```python
from build123d import *

# Parameters (mm, degrees)
SKETCH_1_R          = 7
EXTRUDE_1_DEPTH     = 2
SKETCH_2_W          = 16
SKETCH_2_H          = 16
EXTRUDE_2_DEPTH     = 18
SKETCH_3_W          = 8
SKETCH_3_H          = 16
CUT_EXTRUDE_1_DEPTH = 16
CUT_EXTRUDE_2_DEPTH = 16


with BuildPart() as part:
    # 草图1 → 凸台-拉伸1 (new body)
    with BuildSketch(Plane(origin=(0, 0, 0), x_dir=(1, 0, 0), z_dir=(0, 1, 0))):
        Circle(SKETCH_1_R)
    extrude(amount=EXTRUDE_1_DEPTH)

    # 草图2 → 凸台-拉伸2 (add)
    with BuildSketch(Plane(origin=(0, 2, 0), x_dir=(1, 0, 0), z_dir=(0, 1, 0))):
        Rectangle(SKETCH_2_W, SKETCH_2_H)
    extrude(amount=EXTRUDE_2_DEPTH)

    # 草图3 → 切除-拉伸1 (cut)
    with BuildSketch(Plane.XY.offset(8)):
        with Locations((0, 12)):
            Rectangle(SKETCH_3_W, SKETCH_3_H)
    extrude(amount=-CUT_EXTRUDE_1_DEPTH, mode=Mode.SUBTRACT)

    # 草图4 → 切除-拉伸2 (cut)
    with BuildSketch(Plane(origin=(8, 0, 0), x_dir=(0, 0, -1), z_dir=(1, 0, 0))):
        with BuildLine():
            Line((-8, 12), (-8, 21.557868838))
            Line((-8, 21.557868838), (8, 21.557868838))
            Line((8, 21.557868838), (8, 12))
            ThreePointArc((8, 12), (0, 20), (-8, 12))
        make_face()
    extrude(amount=-CUT_EXTRUDE_2_DEPTH, mode=Mode.SUBTRACT)


solid = part.part
```
The listing builds one solid part. Answer for the finished solid, in the listing's coordinates (mm). A direction names the side the tool comes from. Give positions to 0.01 mm unless a question says otherwise; leave off trailing zeros. Order: outer loops, then holes, each group sorted by start corner. A loop starts at its lowest first (then second) coordinate and runs counter-clockwise, first axis right, second up.
1) Find section D-D on z = -4. Write down the section's boundary in (x, y), then the cut area to 3 significant figures.
Reported:
outline: (-8, 2) - (-5.74, 2) - (-5.74, 0) - (5.74, 0) - (5.74, 2) - (8, 2) - (8, 18.93) - (4, 18.93) - (4, 4) - (-4, 4) - (-4, 18.93) - (-8, 18.93) - close
area: 174 mm2
2) Consider line 1 along X through (y, z) = (16.5, -1.5); line 2 along Y through (x, z) = (0, 3.75); line 3 along Y through (x, z) = (-3.5, 6.5). Determine where each line is inside the solid, lowest interval first.
Reported:
line 1: x = -8 to -4, 4 to 8
line 2: y = 0 to 4
line 3: y = 2 to 4
3) Find section A-A on y = 13.75. Write down the section's boundary in (x, z).
Reported:
outline: (-8, -7.81) - (-4, -7.81) - (-4, 7.81) - (-8, 7.81) - close; (4, -7.81) - (8, -7.81) - (8, 7.81) - (4, 7.81) - close
4) Find section C-C on x = -0.75. Write down the section's boundary in (y, z), then the cut area to 3 significant figures.
Reported:
outline: (0, -6.96) - (2, -6.96) - (2, -8) - (4, -8) - (4, 8) - (2, 8) - (2, 6.96) - (0, 6.96) - close
area: 59.8 mm2
5) Determine the mould class of faces 4 (the face through (4, 12, 0)), 5 (the face through (-0.1, 3.6, 8)), 6 (the face through (0, 4, 0)), 7 (the face through (8, 11, 0)) for opening direction X: pulls with the +X half, pulls with the -X half, needs draft (parallel to the pull), parting line crosses it, or undercut.
Reported:
face 4: undercut
face 5: needs draft
face 6: undercut
face 7: pulls with the +X half
6) For faces 1 (the face through (6, 20, 0)), 2 (the face through (-4, 12, 0)), 3 (the face through (6.466, 0.986, 2.681)), determine the directions among +Z, -Z, +X, -X, +Y, -Y from which every point of the face is accessible in a straight line to the end or side of a thin tool.
Reported:
face 1: +X, -X, +Y
face 2: +Z, -Z, +Y
face 3: -Y
7) Given P1, Ø2, axis at x = -5, z = 3.5, coming from the -Y side; P2, Ø6.5, axis at x = 0, z = -1.5, coming from the +Y side; P3, Ø1, axis at x = -2.5, y = 11.5, coming from the -Z side, each flat-ended and moving along its own axis, determine where each tip first touches the part or whether it passes through.
Reported:
P1: stops at y = 0
P2: stops at y = 4
P3: passes through
8) Find section B-B on z = 0. Write down the section's boundary in (x, y).
Reported:
outline: (-8, 2) - (-7, 2) - (-7, 0) - (7, 0) - (7, 2) - (8, 2) - (8, 20) - (4, 20) - (4, 4) - (-4, 4) - (-4, 20) - (-8, 20) - close
